Work out the finished part from the listing and answer in its coordinate system (mm). A direction names the side the tool comes from. Coordinates: 2 decimals unless noted, no trailing zeros. Loops run counter-clockwise (first coordinate to the right, second up) from the corner with the lowest first, then second, coordinate; pieces in that order, holes last. Notation, with made-up numbers: (15.5, 61.25) -> (49.5, 61.25) arc R31 cw to (49.5, 92.25) -> close; hole circle Ø2 at (12, -25.5). An arc over 180 degrees is marked (long way). One line per question, with ' | ' between items.
```python
from build123d import *

# Parameters (mm, degrees)
F1_DEPTH = 50
F2_R     = 3
F3_DEPTH = 25
F5_R     = 9.5
F5_R_2   = 5
F6_DEPTH = 36


with BuildPart() as f1:
    # F0 (on Front) → F1 (new body)
    with BuildSketch(Plane.XZ):
        with BuildLine():
            Line((0, 9), (0, 0))
            Line((0, 0), (29.635604471, 0))
            ThreePointArc((29.635604471, 0), (24.1372813391, 3.0739592866), (22.0012044628, 9))
            Line((22.0012044628, 9), (0, 9))
        make_face()
        with BuildLine():
            ThreePointArc((22.0012044628, 9), (24.1372813391, 3.0739592866), (29.635604471, 0))
            Line((29.635604471, 0), (32.3655999918, 0))
            ThreePointArc((32.3655999918, 0), (37.7961142893, 2.9949521539), (40, 8.7917712569))
            Line((40, 8.7917712569), (40, 9))
            ThreePointArc((40, 9), (31.0006022314, 17.8958856284), (22.0012044628, 9))
        make_face()
        with BuildLine():
            Line((32.3655999918, 0), (29.635604471, 0))
            ThreePointArc((29.635604471, 0), (31.0006022314, -0.1041143716), (32.3655999918, 0))
        make_face()
        with BuildLine():
            Line((40, 9), (40, 8.7917712569))
            ThreePointArc((40, 8.7917712569), (40.0004516723, 8.8438275718), (40.0006022314, 8.8958856284))
            ThreePointArc((40.0006022314, 8.8958856284), (40.0004516723, 8.9479436851), (40, 9))
        make_face()
    extrude(amount=-F1_DEPTH)

    # F2 (on face) → F3 (cut)
    with BuildSketch(Plane.XY.offset(9)):
        with Locations((11.0006022314, 38)):
            Circle(F2_R)
        with Locations((11.0006022314, 12)):
            Circle(F2_R)
    extrude(amount=-F3_DEPTH, mode=Mode.SUBTRACT)

    # F5 (on offset) → F6 (cut)
    with BuildSketch(Plane.XZ.offset(-7)):
        with Locations((31.0006022314, 8.8958856284)):
            Circle(F5_R)
        with Locations((31.0006022314, 8.8958856284)):
            Circle(F5_R_2, mode=Mode.SUBTRACT)
    extrude(amount=-F6_DEPTH, mode=Mode.SUBTRACT)


solid = f1.part
```
1) Find section D-D (y = 44.5). Write down the section's boundary in (x, z), plus the area to 3 significant figures.
Check values:
outline: (0, 0) -> (29.64, 0) arc R9 ccw (long way) to (22, 9) -> (0, 9) -> close | area: 469 mm^2
2) Find section C-C (z = 6.25). Write down the section's boundary in (x, y), plus the area to 3 significant figures.
Check values:
outline: (0, 0) -> (39.6, 0) -> (39.6, 7) -> (35.24, 7) -> (35.24, 43) -> (39.6, 43) -> (39.6, 50) -> (0, 50) -> close; hole circle Ø6 at (11, 12); hole circle Ø6 at (11, 38); hole (21.88, 7) -> (26.76, 7) -> (26.76, 43) -> (21.88, 43) -> close | area: 1,590 mm^2
3) Find section B-B (z = 2.5). Write down the section's boundary in (x, y), plus the area to 3 significant figures.
Check values:
outline: (0, 0) -> (37.33, 0) -> (37.33, 7) -> (23.98, 7) -> (23.98, 43) -> (37.33, 43) -> (37.33, 50) -> (0, 50) -> close; hole circle Ø6 at (11, 12); hole circle Ø6 at (11, 38) | area: 1,330 mm^2
4) Find section A-A (y = 12). Write down the section's boundary in (x, z), plus the area to 3 significant figures.
Check values:
outline: (0, 0) -> (8, 0) -> (8, 9) -> (0, 9) -> close; (14, 0) -> (27.67, 0) arc R9.5 cw to (21.5, 9) -> (14, 9) -> close; circle Ø10 at (31, 8.9) | area: 233 mm^2
5) The mould has two halves that part along Y. Classify faces 4 (the face through (15, 25, 0)), 5 (the face through (24, 50, 7)), 6 (the face through (35, 7, 5)): released by +Y, released by -Y, zero draft, split by the parting line, or undercut.
Check values:
face 4: zero draft | face 5: released by +Y | face 6: undercut
6) Flat-ended cylindrical pins translate along their axes: pin 1 (24 mm diameter, centred on x = 12.5, y = 26.5, fed in from +Z); pin 2 (7 mm diameter, centred on x = 11, y = 12, fed in from -Z); pin 3 (3.5 mm diameter, centred on x = 11, y = 38, fed in from +Z); pin 4 (2 mm diameter, centred on y = 40.5, z = 12.5, fed in from +X). Find the tip coordinate at first contact, or state that the pin passes through.
Check values:
pin 1: stops at z = 9 | pin 2: stops at z = 0 | pin 3: passes through | pin 4: stops at x = 35.27
7) Find the intervals of material crossed by line 1 along Y through (x, z) = (31.5, 14); line 2 along Y through (x, z) = (12.5, 5); line 3 along Z through (x, y) = (21, 4), in increasing order.
Check values:
line 1: y = 0 to 7, 43 to 50 | line 2: y = 0 to 9.4, 14.6 to 35.4, 40.6 to 50 | line 3: z = 0 to 9
8) For faces 1 (the face through (35, 43, 5)), 2 (the face through (11, 25, 9)), 3 (the face through (24, 0, 7)), determine the directions among +Z, -Z, +X, -X, +Y, -Y from which every point of the face is accessible in a straight line to the end or side of a thin tool.
Check values:
face 1: none | face 2: +Z, -X, +Y, -Y | face 3: +Z, -Z, +X, -X, -Y
